Read the model definition and answer for the solid it produces. Units are mm, in the model's axes. A direction names the side the tool comes from. Round coordinates to 2 decimals unless told otherwise and drop trailing zeros. Order: outer loops, then holes, each group sorted by start corner. A loop starts at its lowest first (then second) coordinate and runs counter-clockwise, first axis right, second up. Notation, with made-up numbers: M 62.25,40.5 L 117.25,40.5 A27 ccw 117.25,71.5 Z; hole C 49.5,-40 d9. An arc over 180 degrees is marked long. Answer as CSV lines item,"result".
Autodesk Inventor part; units mm, degrees
ref_plane "YZ Plane" through (0, 0, 0) normal (1, 0, 0) x (0, 1, 0)
ref_plane "XZ Plane" through (0, 0, 0) normal (0, 1, 0) x (-1, 0, 0)
ref_plane "XY Plane" through (0, 0, 0) normal (0, 0, 1) x (1, 0, 0)
sketch "Sketch1" plane through (0, 0, 0) normal (0, 1, 0) x (-1, 0, 0)
  line L0 (39, -28.5) -> (-39, -28.5)
  line L1 (-39, -28.5) -> (-39, 28.5)
  line L2 (-39, 28.5) -> (39, 28.5)
  line L3 (39, 28.5) -> (39, -28.5)
  line L4 (39, -28.5) -> (-39, 28.5) construction
  line L5 (-39, -28.5) -> (39, 28.5) construction
  point P0 (0, 0)
  dimension "d0" = 78
  dimension "d1" = 57
extrude "Plate1" add sketch "Sketch1" along normal blind 2.5
sketch "Sketch2" plane through (-41.5, 5, 28.5) normal (-1, 0, 0) x (0, -1, 0)
  line L0 (0, -57) -> (0, 0)
  line L1 (0, 0) -> (-58.5, 0)
  line L2 (-58.5, 0) -> (-58.5, -57)
  line L3 (-58.5, -57) -> (0, -57)
edge flange "Flange1" height 63.5 angle 90 thickness 2.5 bend radius 2.5 thickness toward (-1, 0, 0) relief tear relief width 2.5 relief depth 1.25 edges at (-39, 2.5, 0) wall of the first edge with corners at (-41.5, 5, -28.5) (-41.5, 5, 28.5) (-41.5, 63.5, 28.5) (-41.5, 63.5, -28.5)
bend "Bend1"
corner "Corner1"
sketch "Sketch3" plane through (-41.5, 63.5, 28.5) normal (1, 0, 0) x (0, 0, -1)
  line L0 (57, 0) -> (57, -58.5)
  line L1 (0, 0) -> (57, 0)
  line L2 (57, 0) -> (57, -57)
  line L3 (57, -57) -> (0, -57)
  line L4 (0, -57) -> (0, 0)
  line L5 (0, 0) -> (57, -57)
  circle A0 centre (28.5, -28.5) radius 19.25
  line L6 (0, 0) -> (5, 0)
  line L7 (57, 0) -> (0, 0)
  line L8 (5, 0) -> (5, -5)
  line L9 (57, 0) -> (52, 0)
  line L10 (52, 0) -> (52, -5)
  line L11 (57, -57) -> (52, -57)
  line L12 (52, -57) -> (52, -52)
  line L13 (0, -57) -> (5, -57)
  line L14 (5, -57) -> (5, -52)
  circle A1 centre (5, -52) radius 2.5
  circle A2 centre (52, -52) radius 2.5
  circle A3 centre (52, -5) radius 2.5
  circle A4 centre (5, -5) radius 2.5
  point P0 (28.5, -63.5)
  dimension "d13" = 57
  dimension "d14" = 38.5
  dimension "d15" = 5
  dimension "d16" = 5
  dimension "d17" = 5
  dimension "d18" = 5
  dimension "d19" = 5
  dimension "d20" = 5
  dimension "d21" = 5
  dimension "d22" = 5
  dimension "d23" = 5
  dimension "d24" = 5
  dimension "d25" = 5
  dimension "d26" = 5
extrude "Cut1" cut sketch "Sketch3" against normal blind 2.5 contours A2 L12 L5 | L5 A2 | A2 L5 L12 | A4 L5 L8 | L8 L5 A4 | L5 A4 | A0 L5 | L5 A0 | A1 | A3
sketch "Sketch4" plane through (39, 0, -28.5) normal (0, 0, -1) x (-1, 0, 0)
  line L0 (39, 0) -> (29, 0)
  line L1 (78, 0) -> (0, 0)
  line L2 (29, 0) -> (29, 2.5)
  line L3 (78, 2.5) -> (0, 2.5)
  line L4 (29, 2.5) -> (49, 2.5)
  line L5 (49, 2.5) -> (49, 0)
  line L6 (49, 0) -> (29, 0)
  line L7 (29, 0) -> (29, 2.5)
  dimension "d29" = 10
  dimension "d30" = 20
extrude "Extrusion1" add sketch "Sketch4" along normal blind 1
sketch "Sketch5" plane through (-10, 5, -32) normal (0, 0, -1) x (-1, 0, 0)
  line L0 (-20, 0) -> (0, 0)
  line L1 (0, 0) -> (0, 57)
  line L2 (0, 57) -> (-20, 57)
  line L3 (-20, 57) -> (-20, 0)
edge flange "Flange2" height 62 angle 90 thickness 2.5 bend radius 2.5 thickness toward (0, 0, -1) relief tear relief width 2.5 relief depth 1.25 edges at (0, 2.5, -29.5) wall of the first edge with corners at (10, 5, -32) (-10, 5, -32) (-10, 62, -32) (10, 62, -32)
bend "Bend2"
corner "Corner2"
sketch "Sketch6" plane through (-10, 64.5, -29.5) normal (0, 1, 0) x (-1, 0, 0)
  line L0 (-20, 0) -> (0, 0)
  line L1 (0, 0) -> (0, 28)
  line L2 (0, 28) -> (-20, 28)
  line L3 (-20, 28) -> (-20, 0)
edge flange "Flange3" height 33 angle 90 thickness 2.5 bend radius 2.5 thickness toward (0, 1, 0) relief tear relief width 2.5 relief depth 1.25 edges at (0, 62, -32) wall of the first edge with corners at (10, 64.5, -29.5) (-10, 64.5, -29.5) (-10, 64.5, -1.5) (10, 64.5, -1.5)
bend "Bend3"
corner "Corner3"
sketch "Sketch7" plane through (0, 2.5, 0) normal (0, 1, 0) x (1, 0, 0)
  line L0 (39, -28.5) -> (-39, -28.5)
  line L1 (0, -28.5) -> (0, -13.5)
  line L2 (0, -13.5) -> (20, -13.5)
  line L3 (0, -13.5) -> (-20, -13.5)
  circle A0 centre (-20, -13.5) radius 2.25
  circle A1 centre (20, -13.5) radius 2.25
  line L4 (0, -13.5) -> (0, 13.5)
  line L5 (0, 13.5) -> (20, 13.5)
  line L6 (0, 13.5) -> (-20, 13.5)
  circle A2 centre (-20, 13.5) radius 2.25
  circle A3 centre (20, 13.5) radius 2.25
  point P0 (0, 0)
  dimension "d53" = 15
  dimension "d54" = 20
  dimension "d55" = 20
  dimension "d56" = 4.5
  dimension "d57" = 4.5
  dimension "d58" = 27
  dimension "d59" = 20
  dimension "d60" = 20
  dimension "d61" = 4.5
  dimension "d62" = 4.5
extrude "Cut2" cut sketch "Sketch7" against normal blind 2.5
equation "\"d27\" = Thickness"
equation "\"d63\" = Thickness"
equation "\"d3\" = BendReliefWidth"
equation "\"d4\" = BendReliefDepth"
equation "\"d5\" = MinimumRemnant"
equation "\"d6\" = BendRadius"
equation "\"d9\" = BendRadius"
equation "\"d10\" = CornerReliefSize"
equation "\"d11\" = GapSize"
equation "\"d12\" = JacobiRadiusSize"
equation "\"d33\" = BendReliefWidth"
equation "\"d34\" = BendReliefDepth"
equation "\"d35\" = MinimumRemnant"
equation "\"d36\" = BendRadius"
equation "\"d39\" = BendRadius"
equation "\"d40\" = CornerReliefSize"
equation "\"d41\" = GapSize"
equation "\"d42\" = JacobiRadiusSize"
equation "\"d43\" = BendReliefWidth"
equation "\"d44\" = BendReliefDepth"
equation "\"d45\" = MinimumRemnant"
equation "\"d46\" = BendRadius"
equation "\"d49\" = BendRadius"
equation "\"d50\" = CornerReliefSize"
equation "\"d51\" = GapSize"
equation "\"d52\" = JacobiRadiusSize"
equation "\"BendRadius\" = Thickness"
equation "\"BendReliefWidth\" = Thickness"
equation "\"BendReliefDepth\" = 0.5 * Thickness"
equation "\"MinimumRemnant\" = 2 * Thickness"
equation "\"TransitionRadius\" = BendRadius"
equation "\"JacobiRadiusSize\" = BendRadius"
equation "\"GapSize\" = Thickness"
equation "\"d2\" = BendRadius"
properties part number "MotorClamptwo" material "Steel, Mild"
Item 1: Find the intervals of material crossed by probe 1 along Z at (x, y) = (-42.9, 11.5); probe 2 along Z at (x, y) = (20, 0.6); probe 3 along Y at (x, z) = (-42, 23), in increasing order. Write a range as [from, to].
Ans:
probe 1,"[-28.5, -26], [-21, 21], [26, 28.5]"
probe 2,"[-28.5, -15.75], [-11.25, 11.25], [15.75, 28.5]"
probe 3,"[1, 9.05], [13.95, 56.05], [60.95, 63.5]"
Item 2: A cutting plane is placed at A-A, the plane x = -20. Determine the outline of the cut face in (y, z), and give its area (3 significant figures).
Ans:
outline,"M 0,-28.5 L 2.5,-28.5 L 2.5,-15.75 L 0,-15.75 Z; M 0,-11.25 L 2.5,-11.25 L 2.5,11.25 L 0,11.25 Z; M 0,15.75 L 2.5,15.75 L 2.5,28.5 L 0,28.5 Z"
area,"120 mm2"
Item 3: A cutting plane is placed at D-D, the plane y = 44.5. Determine the outline of the cut face in (x, z).
Ans:
outline,"M -44,-28.5 L -41.5,-28.5 L -41.5,-16.74 L -44,-16.74 Z; M -44,16.74 L -41.5,16.74 L -41.5,28.5 L -44,28.5 Z; M -10,-34.5 L 10,-34.5 L 10,-32 L -10,-32 Z"
Item 4: A cutting plane is placed at C-C, the plane z = 0. Determine the outline of the cut face in (x, y).
Ans:
outline,"M -44,5 A5 ccw -39,0 L 39,0 L 39,2.5 L -39,2.5 A2.5 cw -41.5,5 L -41.5,15.75 L -44,15.75 Z; M -44,54.25 L -41.5,54.25 L -41.5,63.5 L -44,63.5 Z"
Item 5: Determine the mould class of faces 5 (the face through (-17.854, 1.268, -14.176)), 6 (the face through (-10, 44, -33)), 7 (the face through (-0.14, 1.5, -33.07)) for opening direction X: +X half, -X half, draft (parallel to the pull), parting line (faces both ways), or undercut.
Ans:
face 5,"undercut"
face 6,"-X half"
face 7,"draft"
Item 6: A tool of negligible diameter and unlimited length cuts with its end or side. For faces 1 (the face through (24, 1, -28.5)), 2 (the face through (0, 64, -31)), 3 (the face through (1, 2.5, 0)), 4 (the face through (-42, 22, -28.5)), from which of +Z, -Z, +X, -X, +Y, -Y can it reach the whole face along a straight path? Write none if from no direction.
Ans:
face 1,"-Z, +X, +Y, -Y"
face 2,"+Z, +X, -X"
face 3,"+Z, +X"
face 4,"-Z, -X, +Y, -Y"
Item 7: A cutting plane is placed at B-B, the plane y = 11.5. Determine the outline of the cut face in (x, z), and give its area (4 significant figures).
Ans:
outline,"M -44,-28.5 L -41.5,-28.5 L -41.5,-26 L -44,-26 Z; M -44,-21 L -41.5,-21 L -41.5,21 L -44,21 Z; M -44,26 L -41.5,26 L -41.5,28.5 L -44,28.5 Z; M -10,-34.5 L 10,-34.5 L 10,-32 L -10,-32 Z"
area,"167.5 mm2"
Item 8: Flat-ended cylindrical pins translate along their axes: pin 1 (12 mm diameter, centred on y = 41, z = -5, fed in from -X); pin 2 (10 mm diameter, centred on y = 25.5, z = -21.5, fed in from +X); pin 3 (1.2 mm diameter, centred on x = 3, y = 65.5, fed in from +Z); pin 4 (6 mm diameter, centred on x = -20, z = 13.5, fed in from +Y). Find the tip coordinate at first contact, or state that the pin passes through.
Ans:
pin 1,"through"
pin 2,"x = -41.5"
pin 3,"z = -1.5"
pin 4,"y = 2.5"
